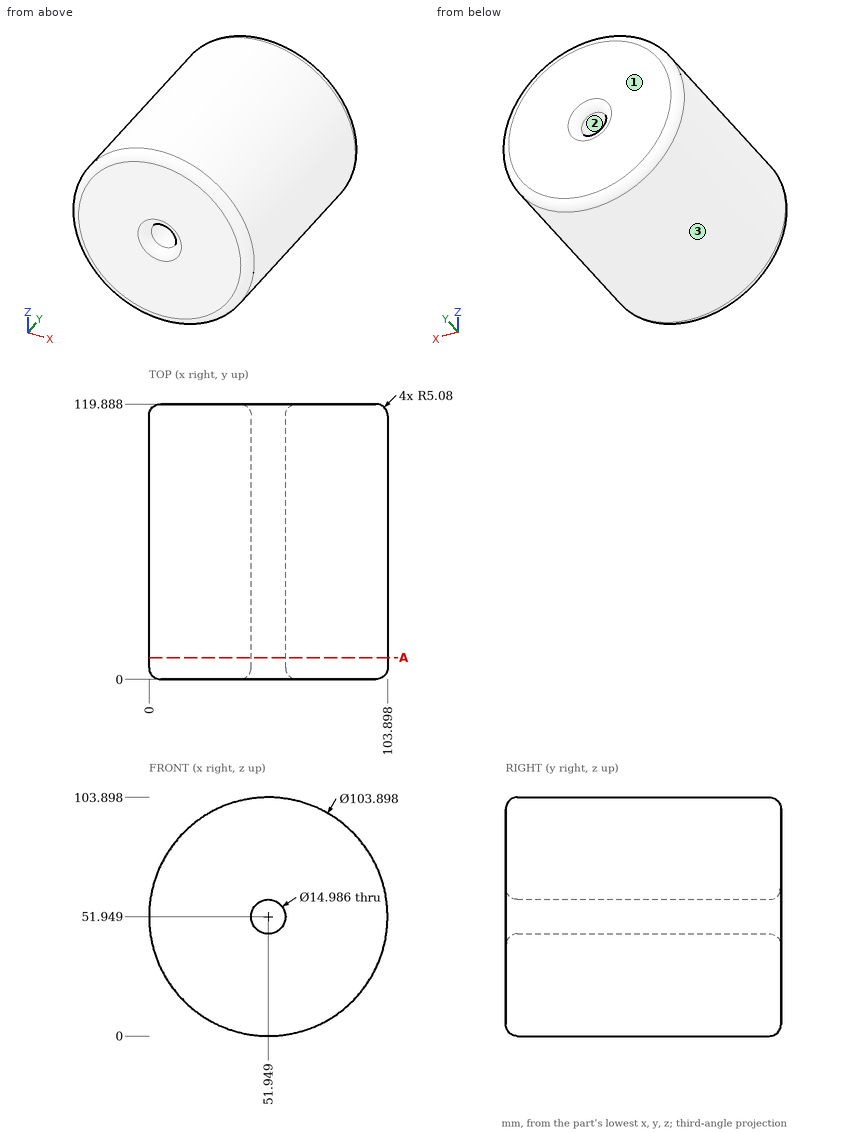
Can you work these out from the drawing? Everything is in mm from the part's minimum corner. Give positions to 0.01 mm unless a question says otherwise; leave off trailing zeros. Loops run counter-clockwise (first coordinate to the right, second up) from the corner with the lowest first, then second, coordinate; pieces in that order, holes last. Notation, with made-up numbers: (27, 78) - (70, 78) arc R10 cw to (70, 93) - close; hole circle Ø7 at (-16.5, 53). An arc over 180 degrees is marked (long way). Use one line per item in the form item = value.
1. I need wall thicknesses on probe 1 along Z at (x, y) = (53, 89); probe 2 along X at (y, z) = (36, 54) (1 decimal). Which ranges of each line are inside material? Lowest first, please.
Response values:
probe_1 = 0.01 to 44.53, 59.37 to 103.89
probe_2 = 0 to 44.7, 59.2 to 103.9
2. Thinking about a two-plate mould opening in X: for the marked faces 1, 2 and 3, which applies, released by +X, released by -X, zero draft, split by the parting line, or undercut?
Response values:
face_1 = zero draft
face_2 = undercut
face_3 = split by the parting line
3. I'm going to push flat-ended pins straight in: pin 1 Ø4 at (x, y) = (66.5, 26) entering from +Z; pin 2 Ø10 at (y, z) = (57, 17) entering from -X; pin 3 Ø5 at (x, y) = (25, 79.5) entering from +Z (1 decimal). Where does each tip first touch, or does it pass through?
Response values:
pin_1 = 102.36
pin_2 = 9.5
pin_3 = 97.8
4. I want a section at A-A (y = 9.5). Please give me the cut outline in (x, z), and give its area (3 significant figures).
Response values:
outline = circle Ø103.9 at (51.95, 51.95); hole circle Ø14.99 at (51.95, 51.95)
area = 8,300 mm²
